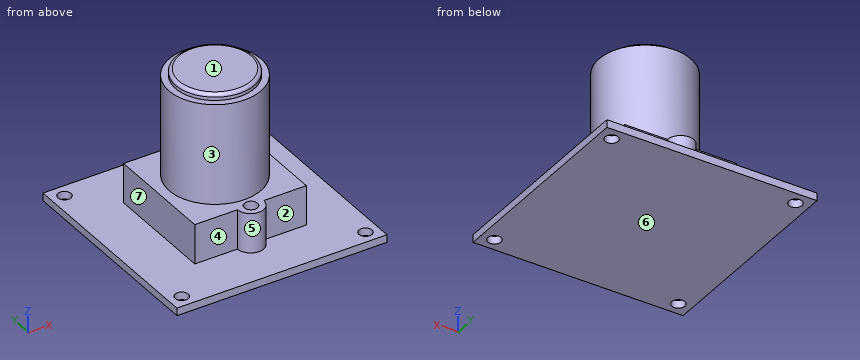
```python
from build123d import *

# Parameters (mm, degrees)
SKETCH1_R           = 7
BOSS_EXTRUDE1_DEPTH = 15.3
SKETCH2_R           = 6
BOSS_EXTRUDE2_DEPTH = 1
FILLET1_R           = 0.5
SKETCH3_W           = 1.163915396
SKETCH3_H           = 32
BOSS_EXTRUDE3_DEPTH = 16
SKETCH4_W           = 17
SKETCH4_H           = 17
BOSS_EXTRUDE4_DEPTH = 6.036084604
SKETCH5_R           = 1
CUT_EXTRUDE1_DEPTH  = 4
SKETCH6_R           = 2
BOSS_EXTRUDE5_DEPTH = 6.036084604
SKETCH7_R           = 0.995331294
SKETCH7_R_2         = 1.011185122
CUT_EXTRUDE2_DEPTH  = 4


with BuildPart() as part:
    # Sketch1 → Boss-Extrude1 (new body)
    with BuildSketch(Plane.XY):
        Circle(SKETCH1_R)
    extrude(amount=BOSS_EXTRUDE1_DEPTH)

    # Sketch2 → Boss-Extrude2 (add)
    with BuildSketch(Plane.XY.offset(15.3)):
        Circle(SKETCH2_R)
    extrude(amount=BOSS_EXTRUDE2_DEPTH)

    # Fillet1
    fillet1_edges = [part.edges().sort_by_distance(p)[0] for p in [
        (-6, 0, 16.3),
    ]]
    fillet(fillet1_edges, radius=FILLET1_R)



with BuildPart() as body_2:
    # Sketch3 → Boss-Extrude3 (new, symmetric)
    with BuildSketch(Plane(origin=(0, 0, 0), x_dir=(0, 0, -1), z_dir=(1, 0, 0))):
        with Locations((6.618042302, 0)):
            Rectangle(SKETCH3_W, SKETCH3_H)
    extrude(amount=BOSS_EXTRUDE3_DEPTH, both=True)


with BuildPart() as part_1:
    add(part.part)

    add(body_2.part)  # Boss-Extrude4 merges body 2
    # Sketch4 → Boss-Extrude4 (add)
    with BuildSketch(Plane.XY.offset(-6.036084604)):
        Rectangle(SKETCH4_W, SKETCH4_H)
    extrude(amount=BOSS_EXTRUDE4_DEPTH)

    # Sketch5 → Cut-Extrude1 (cut)
    with BuildSketch(Plane.XY.offset(-6.036084604)):
        with Locations((-14, 14)):
            Circle(SKETCH5_R)
        with Locations((14, 14)):
            Circle(SKETCH5_R)
        with Locations((14, -14)):
            Circle(SKETCH5_R)
        with Locations((-14, -14)):
            Circle(SKETCH5_R)
    extrude(amount=-CUT_EXTRUDE1_DEPTH, mode=Mode.SUBTRACT)

    # Sketch6 → Boss-Extrude5 (add)
    with BuildSketch(Plane.XY):
        with Locations((0, 8.5)):
            Circle(SKETCH6_R)
        with Locations((0, -8.5)):
            Circle(SKETCH6_R)
    extrude(amount=-BOSS_EXTRUDE5_DEPTH)

    # Sketch7 → Cut-Extrude2 (cut)
    with BuildSketch(Plane.XY):
        with Locations((0, 8.595073535)):
            Circle(SKETCH7_R)
        with Locations((0, -8.595073535)):
            Circle(SKETCH7_R_2)
    extrude(amount=-CUT_EXTRUDE2_DEPTH, mode=Mode.SUBTRACT)


solid = part_1.part
```
Work out the finished part from the listing and answer in its coordinate system (mm). Face numbers are marked on the shaded views. A direction names the side the tool comes from. Coordinates: 2 decimals unless noted, no trailing zeros. Order: outer loops, then holes, each group sorted by start corner. A loop starts at its lowest first (then second) coordinate and runs counter-clockwise, first axis right, second up. Notation, with made-up numbers: (38, 68) - (90, 68) arc R16 cw to (90, 84) - close; hole circle Ø4 at (-14.5, 24). An arc over 180 degrees is marked (long way). Answer as a JSON object with one key per item and string values.
1. Find section C-C on y = 0. Determine the outline of the cut face in (x, z), plus the area to 3 significant figures.
Output values:
{"outline": "(-16, -7.2) - (16, -7.2) - (16, -6.04) - (8.5, -6.04) - (8.5, 0) - (7, 0) - (7, 15.3) - (6, 15.3) - (6, 15.8) arc R0.5 ccw to (5.5, 16.3) - (-5.5, 16.3) arc R0.5 ccw to (-6, 15.8) - (-6, 15.3) - (-7, 15.3) - (-7, 0) - (-8.5, 0) - (-8.5, -6.04) - (-16, -6.04) - close", "area": "366 mm²"}
2. Consider line 1 (Y direction, x = 14, z = -6.25); line 2 (Y direction, x = 0, z = -2.4); line 3 (Z direction, x = -6, y = -13.5). Determine where each line is inside the solid, lowest interval first.
Output values:
{"line 1": "y = -16 to -15, -13 to 13, 15 to 16", "line 2": "y = -10.5 to -9.61, -7.58 to 7.6, 9.59 to 10.5", "line 3": "z = -7.2 to -6.04"}
3. The mould has two halves that part along X. Classify the marked faces 5, 6 and 7: +X half, -X half, draft (parallel to the pull), parting line (faces both ways), or undercut.
Output values:
{"face 5": "parting line", "face 6": "draft", "face 7": "-X half"}
4. Find section A-A on x = 14. Determine the outline of the cut face in (y, z).
Output values:
{"outline": "(-16, -7.2) - (-15, -7.2) - (-15, -6.04) - (-16, -6.04) - close; (-13, -7.2) - (13, -7.2) - (13, -6.04) - (-13, -6.04) - close; (15, -7.2) - (16, -7.2) - (16, -6.04) - (15, -6.04) - close"}
5. Find section D-D on x = 0. Determine the outline of the cut face in (y, z), plus the area to 3 significant figures.
Output values:
{"outline": "(-16, -7.2) - (16, -7.2) - (16, -6.04) - (10.5, -6.04) - (10.5, 0) - (9.59, 0) - (9.59, -4) - (7.6, -4) - (7.6, 0) - (7, 0) - (7, 15.3) - (6, 15.3) - (6, 15.8) arc R0.5 ccw to (5.5, 16.3) - (-5.5, 16.3) arc R0.5 ccw to (-6, 15.8) - (-6, 15.3) - (-7, 15.3) - (-7, 0) - (-7.58, 0) - (-7.58, -4) - (-9.61, -4) - (-9.61, 0) - (-10.5, 0) - (-10.5, -6.04) - (-16, -6.04) - close", "area": "374 mm²"}
6. A tool of negligible diameter and unlimited length cuts with its end or side. For the marked faces 1, 2, 3 and 4, from which of +Z, -Z, +X, -X, +Y, -Y can it reach the whole face along a straight path? Write none if from no direction.
Output values:
{"face 1": "+Z, +X, -X, +Y, -Y", "face 2": "+Z, +X, -Y", "face 3": "+Z", "face 4": "+Z, -X, -Y"}
7. Each of these flat-tipped pins is pushed along its axis until it touches: P1, Ø13.5, axis at x = 3.5, y = -5, coming from the +Z side; P2, Ø0.6, axis at x = 0, y = 9, coming from the +Z side; P3, Ø6.5, axis at x = 5.5, z = -2.5, coming from the -Y side; P4, Ø6, axis at x = 0.5, z = 1, coming from the +Y side. Where does it stop, or does it pass through?
Output values:
{"P1": "stops at z = 16.3", "P2": "stops at z = -4", "P3": "stops at y = -8.5", "P4": "stops at y = 10.5"}
